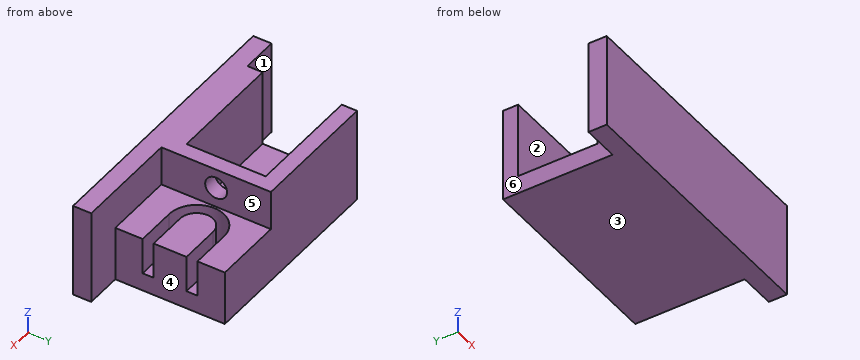
from build123d import *

# Parameters (mm, degrees)
PAD_DEPTH       = 15.5
SKETCH001_W     = 11.5
SKETCH001_H     = 18
POCKET_DEPTH    = 6.5
SKETCH002_W     = 28.698795
SKETCH002_H     = 13
POCKET001_DEPTH = 12.5
SKETCH003_R     = 1.8
POCKET002_DEPTH = 2.5
POCKET003_DEPTH = 6


with BuildPart() as part:
    # Sketch → Pad (new body)
    with BuildSketch(Plane.XY):
        Polygon((-16.5, 3), (-22.5, 3), (-22.5, 0), (22.5, 0), (22.5, 3), (16.5, 3), (16.5, 21), (-16.5, 21), align=None)
    extrude(amount=PAD_DEPTH)

    # Sketch001 → Pocket (cut)
    with BuildSketch(Plane.XY.offset(15.5)):
        with Locations((10.75, 12)):
            Rectangle(SKETCH001_W, SKETCH001_H)
    extrude(amount=-POCKET_DEPTH, mode=Mode.SUBTRACT)

    # Sketch002 → Pocket001 (cut)
    with BuildSketch(Plane.XY.offset(15.5)):
        with Locations((-11.8493975, 12)):
            Rectangle(SKETCH002_W, SKETCH002_H)
    extrude(amount=-POCKET001_DEPTH, mode=Mode.SUBTRACT)

    # Sketch003 → Pocket002 (cut)
    with BuildSketch(Plane(origin=(2.5, 0, 0), x_dir=(0, -1, 0), z_dir=(-1, 0, 0))):
        with Locations((-12, 12.3)):
            Circle(SKETCH003_R)
    extrude(amount=-POCKET002_DEPTH, mode=Mode.SUBTRACT)

    # Sketch004 → Pocket003 (cut)
    with BuildSketch(Plane.XY.offset(9)):
        with BuildLine():
            ThreePointArc((9.8823500905, 16.5019904992), (5.3803595914, 12), (9.8823500905, 7.4980095008))
            Line((9.8823500905, 7.4980095008), (17.636722355, 7.4980095008))
            Line((17.636722355, 9.2980095008), (17.636722355, 7.4980095008))
            Line((9.8823500905, 9.2980095008), (17.636722355, 9.2980095008))
            ThreePointArc((9.8823500905, 14.7019904992), (7.1803595914, 12), (9.8823500905, 9.2980095008))
            Line((9.8823500905, 14.7019904992), (17.636722355, 14.7019904992))
            Line((17.636722355, 16.5019904992), (17.636722355, 14.7019904992))
            Line((9.8823500905, 16.5019904992), (17.636722355, 16.5019904992))
        make_face()
    extrude(amount=-POCKET003_DEPTH, mode=Mode.SUBTRACT)


solid = part.part
Geometry check sheet. Reference: the model listing, model coordinates, mm. Face numbers are marked on the shaded views. A direction names the side the tool comes from. Coordinates: 2 decimals unless noted, no trailing zeros. Order: outer loops, then holes, each group sorted by start corner. A loop starts at its lowest first (then second) coordinate and runs counter-clockwise, first axis right, second up. Notation, with made-up numbers: (62, 0) - (119, 0) arc R12 ccw to (119, 14) - close; hole circle Ø9 at (48, 28.5). An arc over 180 degrees is marked (long way). One line per item, written item: value.
(1) Access from +Z, -Z, +X, -X, +Y, -Y to the whole of each face (thin tool, end or side, straight path). Record for the marked faces 4, 5 and 6.
Data:
face 4: +Z, -Z, +X, +Y
face 5: +Z, +X, +Y
face 6: +Z, -Z, -X, +Y
(2) Sectioned sample at A-A (y = 12). Enter the section's corners in (x, z).
Data:
outline: (-16.5, 0) - (16.5, 0) - (16.5, 9) - (7.18, 9) - (7.18, 3) - (5.38, 3) - (5.38, 9) - (5, 9) - (5, 10.5) - (2.5, 10.5) - (2.5, 3) - (-16.5, 3) - close; (2.5, 14.1) - (5, 14.1) - (5, 15.5) - (2.5, 15.5) - close
(3) Sectioned sample at D-D (y = 6). Enter the section's corners in (x, z).
Data:
outline: (-16.5, 0) - (16.5, 0) - (16.5, 9) - (5, 9) - (5, 15.5) - (2.5, 15.5) - (2.5, 3) - (-16.5, 3) - close
(4) Sectioned sample at C-C (x = 2). Enter the section's corners in (y, z).
Data:
outline: (0, 0) - (21, 0) - (21, 15.5) - (18.5, 15.5) - (18.5, 3) - (5.5, 3) - (5.5, 15.5) - (0, 15.5) - close
(5) Sectioned sample at B-B (z = 12.3). Enter the section's corners in (x, y), and give its area (3 significant figures).
Data:
outline: (-22.5, 0) - (22.5, 0) - (22.5, 3) - (5, 3) - (5, 10.2) - (2.5, 10.2) - (2.5, 5.5) - (-16.5, 5.5) - (-16.5, 3) - (-22.5, 3) - close; (-16.5, 18.5) - (2.5, 18.5) - (2.5, 13.8) - (5, 13.8) - (5, 21) - (-16.5, 21) - close
area: 266 mm^2
(6) Release check for a two-part mould opening along Y. For the marked faces 1, 2 and 3 record: +Y half, -Y half, draft (parallel to the pull), parting line (faces both ways), or undercut.
Data:
face 1: +Y half
face 2: undercut
face 3: draft
(7) Depth check by flat-ended pin: pin 1 Ø6 at (y, z) = (19, 4) entering from +X; pin 2 Ø3 at (y, z) = (12, 12.3) entering from -X; pin 3 Ø4.5 at (y, z) = (8, 8) entering from -X; pin 4 Ø2 at (y, z) = (18, 9.5) entering from -X. Enter the tip coordinate at first touch or a pass-through.
Data:
pin 1: stops at x = 16.5
pin 2: passes through
pin 3: stops at x = 2.5
pin 4: stops at x = -16.5
(8) Thickness scan on probe 1 along Y at (x, z) = (-13, 11.5); probe 2 along Z at (x, y) = (4.2, 12); probe 3 along X at (y, z) = (3.5, 1). Record the ranges inside material, lowest first. Write a range as from..to.
Data:
probe 1: y = 0..5.5, 18.5..21
probe 2: z = 0..10.5, 14.1..15.5
probe 3: x = -16.5..16.5
